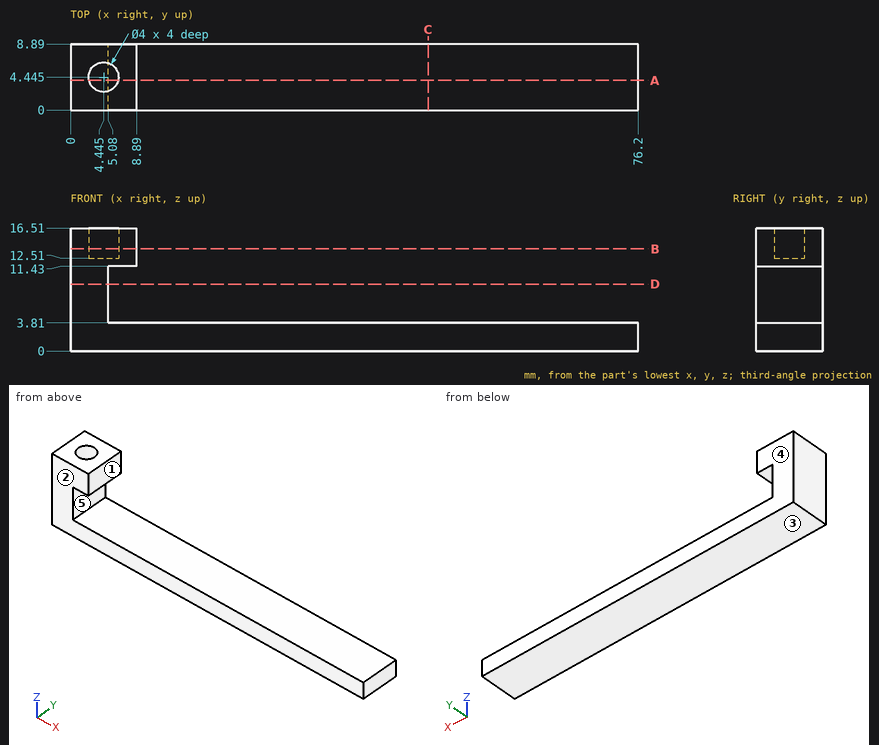
Drawing for the job (mm, zero at the part's lowest x, y, z). A direction names the side the tool comes from. Round coordinates to 2 decimals unless told otherwise and drop trailing zeros. Write each loop counter-clockwise with the first axis right and the second up, starting at its lowest first coordinate (ties: lowest second). Pieces come first, ordered by that corner, then holes. Notation, with made-up numbers: (-14, -30.75) - (8, -30.75) arc R11 cw to (8, -13.75) - close; hole circle Ø7 at (67, 59.5). An arc over 180 degrees is marked (long way). Write item = value, one per line. Start each with the question number.
Q1. Drop flat-ended pins along their axis: pin 1 (5 mm diameter, centred on y = 1, z = 7, fed in from -X); pin 2 (4 mm diameter, centred on x = 53, y = 3.5, fed in from +Z); pin 3 (4 mm diameter, centred on y = 3.5, z = 6.5, fed in from +X). Give the stop position or say it passes through.
Q2. Which spindle directions (+Z, -Z, +X, -X, +Y, -Y) get a long thin tool onto all of the face, cutting with end or side? Do the marked faces 1 and 2. Say none if no direction does.
Q3. Band-saw the part on D-D (z = 9). Give the cut face in (x, y), then the cut area to 3 significant figures.
Q4. Band-saw the part on A-A (y = 4). Give the cut face in (x, z).
Q5. Probe L1, parallel to X at y = 4.5, z = 15.5; L2, parallel to Z at x = 8, y = 4; L3, parallel to X at y = 1.5, z = 10. List the from-to ranges inside material, lowest first. Write a range as from..to.
Q6. Mould opens along Z. For the marked faces 3, 4 and 5 say: pulls with the +Z half, pulls with the -Z half, needs draft (parallel to the pull), parting line crosses it, or undercut.
Q7. Band-saw the part on B-B (z = 13.75). Give the cut face in (x, y) (3 decimals).
Q8. Band-saw the part on C-C (x = 48). Give the cut face in (y, z).
Answers below:
q1.pin_1 = 0
q1.pin_2 = 3.81
q1.pin_3 = 5.08
q2.face_1 = +Z, +X, +Y, -Y
q2.face_2 = +Z, -Z, +X, -X, -Y
q3.outline = (0, 0) - (5.08, 0) - (5.08, 8.89) - (0, 8.89) - close
q3.area = 45.2 mm2
q4.outline = (0, 0) - (76.2, 0) - (76.2, 3.81) - (5.08, 3.81) - (5.08, 11.43) - (8.89, 11.43) - (8.89, 16.51) - (6.39, 16.51) - (6.39, 12.51) - (2.5, 12.51) - (2.5, 16.51) - (0, 16.51) - close
q5.L1 = 0..2.45, 6.44..8.89
q5.L2 = 0..3.81, 11.43..16.51
q5.L3 = 0..5.08
q6.face_3 = pulls with the -Z half
q6.face_4 = needs draft
q6.face_5 = undercut
q7.outline = (0, 0) - (8.89, 0) - (8.89, 8.89) - (0, 8.89) - close; hole circle Ø4 at (4.445, 4.445)
q8.outline = (0, 0) - (8.89, 0) - (8.89, 3.81) - (0, 3.81) - close
